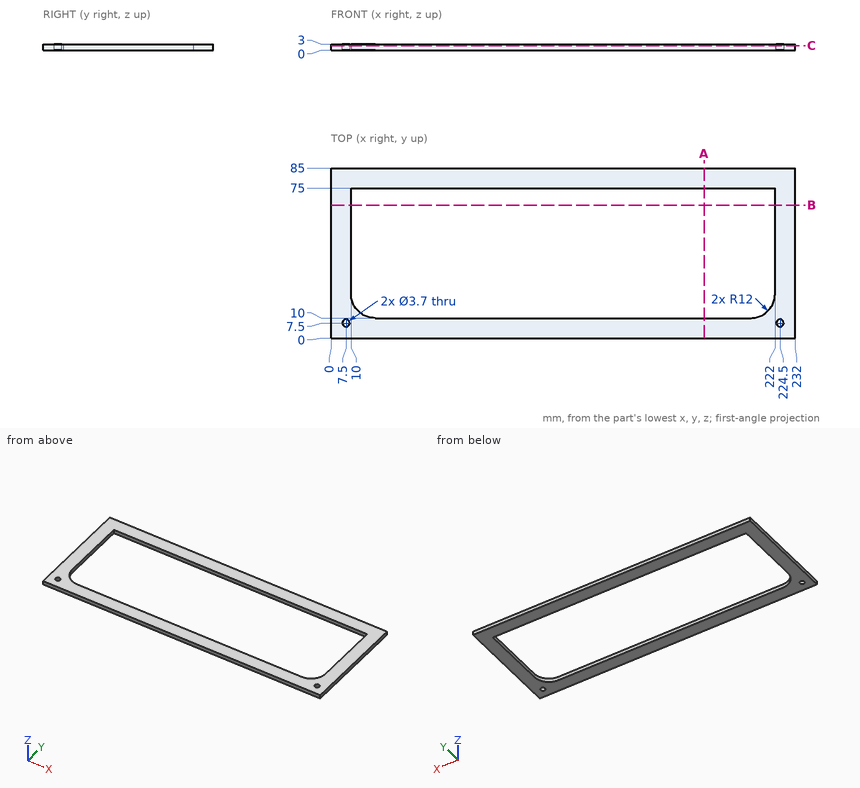
Verification items for this drawing (mm, ordinates from the low corner). Give positions to 0.01 mm unless a question says otherwise; leave off trailing zeros. Loops run counter-clockwise (first coordinate to the right, second up) from the corner with the lowest first, then second, coordinate; pieces in that order, holes last. Notation, with made-up numbers: M 73,-3 L 121,-3 A16 ccw 121,3 Z; hole C 35.25,-32 d3. An arc over 180 degrees is marked long. Answer as CSV lines item,"result".
Item 1: Cross-section at C-C on z = 2.2. Record the cut outline in (x, y).
Values:
outline,"M 0,0 L 232,0 L 232,85 L 0,85 Z; hole C 7.5,7.5 d3.7; hole M 10,22 A12 ccw 22,10 L 210,10 A12 ccw 222,22 L 222,75 L 10,75 Z; hole C 224.5,7.5 d3.7"
Item 2: Cross-section at B-B on y = 66.5. Record the cut outline in (x, z), and give its area (3 significant figures).
Values:
outline,"M 0,0 L 10,0 L 10,3 L 0,3 Z; M 222,0 L 232,0 L 232,3 L 222,3 Z"
area,"60.0 mm²"
Item 3: Cross-section at A-A on x = 186.5. Record the cut outline in (y, z), and give its area (3 significant figures).
Values:
outline,"M 0,0 L 10,0 L 10,3 L 0,3 Z; M 75,0 L 85,0 L 85,3 L 75,3 Z"
area,"60.0 mm²"
Item 4: Depth check by flat-ended pin: P1, Ø1.5, axis at x = 135, z = 1, coming from the -Y side. Enter the tip coordinate at first touch or a pass-through.
Values:
P1,"stops at y = 0"
Item 5: Material ranges on line 1 (Y direction, x = 54.5, z = 0.5); line 2 (Y direction, x = 7.5, z = 1.45); line 3 (X direction, y = 36, z = 1.65), recorded low to high.
Values:
line 1,"y = 0 to 10, 75 to 85"
line 2,"y = 0 to 5.65, 9.35 to 85"
line 3,"x = 0 to 10, 222 to 232"
